The model under review builds one solid part; all positions refer to its coordinate system, in mm. Face numbers are marked on the shaded views. A direction names the side the tool comes from. Coordinates: 2 decimals unless noted, no trailing zeros. Loops run counter-clockwise (first coordinate to the right, second up) from the corner with the lowest first, then second, coordinate; pieces in that order, holes last. Notation, with made-up numbers: (38, 23.5) - (69, 23.5) arc R28 cw to (69, 56.5) - close; hole circle Ø7 at (72.25, 25.25). An arc over 180 degrees is marked (long way). Answer in a Markdown table with one row per item. Add a question column.
(1) Mouldability with a two-part tool opening along Z and no side actions: class the marked faces 1, 2 and 3 as +Z half, -Z half, draft (parallel to the pull), parting line (faces both ways), or undercut.
(2) For P1, Ø2, axis at x = -1.5, y = 0.5, coming from the +Z side; P2, Ø3, axis at x = -2, y = -0.5, coming from the -Z side; P3, Ø2, axis at y = 0.5, z = 4, coming from the -X side, all flat-tipped, find the tip position at first contact; note any pin that passes through.
(3) We need section C-C on y = 1.55. Write out the cut boundary in (x, z).
(4) We need section A-A on z = 0. Write out the cut boundary in (x, y).
(5) Machinability: for the marked faces 4, 5 and 6, which of the approach directions +Z, -Z, +X, -X, +Y, -Y give a long, thin tool a straight path to every point of the face, cutting with its end or side? Answer none if there is none.
(6) We need section D-D on x = -3.5. Write out the cut boundary in (y, z), plus the area to 3 significant figures.
(7) We need section B-B on x = 0. Write out the cut boundary in (y, z).
(8) For line 1 along Z through (x, y) = (0, -2.05); line 2 along Z through (x, y) = (0, 1.2), list the stretches that pass through material, from the lowest coordinate up.
from build123d import *

# Parameters (mm, degrees)
SKETCH1_R           = 8
SKETCH1_R_2         = 2.5
BOSS_EXTRUDE1_DEPTH = 2.5
SKETCH2_R           = 6.5
SKETCH2_R_2         = 4
CUT_EXTRUDE1_DEPTH  = 0.5
CHAMFER1_SIZE       = 0.1


with BuildPart() as part:
    # Sketch1 → Boss-Extrude1 (new body, symmetric)
    with BuildSketch(Plane(origin=(0, 0, 0), x_dir=(1, 0, 0), z_dir=(0, 1, 0))):
        Circle(SKETCH1_R)
        Circle(SKETCH1_R_2, mode=Mode.SUBTRACT)
    extrude(amount=BOSS_EXTRUDE1_DEPTH, both=True)

    # Sketch2 → Cut-Extrude1 (cut)
    with BuildSketch(Plane(origin=(0, 2.5, 0), x_dir=(1, 0, 0), z_dir=(0, 1, 0))):
        Circle(SKETCH2_R)
        Circle(SKETCH2_R_2, mode=Mode.SUBTRACT)
    cut_extrude1 = extrude(amount=-CUT_EXTRUDE1_DEPTH, mode=Mode.SUBTRACT)

    # Mirror1: Cut-Extrude1 across plane
    add(cut_extrude1.mirror(Plane.ZX), mode=Mode.SUBTRACT)

    # Chamfer1
    chamfer1_edges = [part.edges().sort_by_distance(p)[0] for p in [
        (-2.5, -2.5, 0),
        (-2.5, 2.5, 0),
    ]]
    chamfer(chamfer1_edges, length=CHAMFER1_SIZE)


solid = part.part
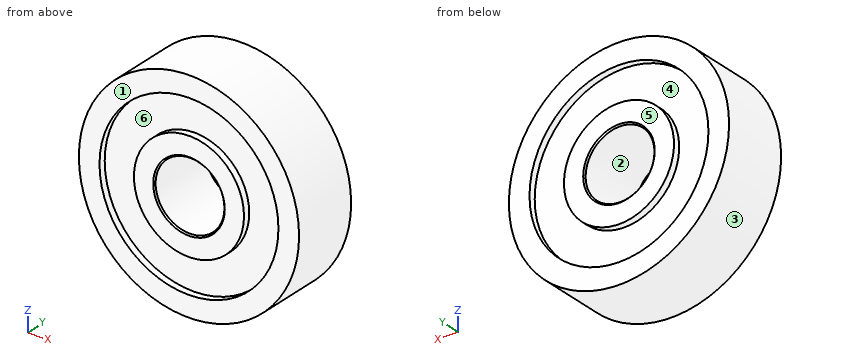
Outcome:
| question | item | result |
|---|---|---|
| 1 | face 1 | draft |
| 1 | face 2 | undercut |
| 1 | face 3 | parting line |
| 2 | P1 | z = 7.98 |
| 2 | P2 | z = -7.98 |
| 2 | P3 | x = -7.42 |
| 3 | outline | circle Ø16 at (0, 0); hole circle Ø5 at (0, 0) |
| 4 | outline | (-8, -2.5) - (-6.5, -2.5) - (-6.5, -2) - (-4, -2) - (-4, -2.5) - (-2.6, -2.5) - (-2.5, -2.4) - (-2.5, 2.4) - (-2.6, 2.5) - (-4, 2.5) - (-4, 2) - (-6.5, 2) - (-6.5, 2.5) - (-8, 2.5) - close; (2.5, -2.4) - (2.6, -2.5) - (4, -2.5) - (4, -2) - (6.5, -2) - (6.5, -2.5) - (8, -2.5) - (8, 2.5) - (6.5, 2.5) - (6.5, 2) - (4, 2) - (4, 2.5) - (2.6, 2.5) - (2.5, 2.4) - close |
| 5 | face 4 | +Y |
| 5 | face 5 | +Z, -Z, +X, -X, +Y |
| 5 | face 6 | -Y |
| 6 | outline | (-2.5, -7.19) - (2.5, -7.19) - (2.5, -5.48) - (2, -5.48) - (2, -1.94) - (2.5, -1.94) - (2.5, 1.94) - (2, 1.94) - (2, 5.48) - (2.5, 5.48) - (2.5, 7.19) - (-2.5, 7.19) - (-2.5, 5.48) - (-2, 5.48) - (-2, 1.94) - (-2.5, 1.94) - (-2.5, -1.94) - (-2, -1.94) - (-2, -5.48) - (-2.5, -5.48) - close |
| 6 | area | 64.9 mm² |
| 7 | outline | (-2.5, -8) - (2.5, -8) - (2.5, -6.5) - (2, -6.5) - (2, -4) - (2.5, -4) - (2.5, -2.6) - (2.4, -2.5) - (-2.4, -2.5) - (-2.5, -2.6) - (-2.5, -4) - (-2, -4) - (-2, -6.5) - (-2.5, -6.5) - close; (-2.5, 2.6) - (-2.4, 2.5) - (2.4, 2.5) - (2.5, 2.6) - (2.5, 4) - (2, 4) - (2, 6.5) - (2.5, 6.5) - (2.5, 8) - (-2.5, 8) - (-2.5, 6.5) - (-2, 6.5) - (-2, 4) - (-2.5, 4) - close |
| 8 | line 1 | -8 to -6.5, -4 to -2.5, 2.5 to 4, 6.5 to 8 |
| 8 | line 2 | -8 to -2.5, 2.5 to 8 |
